Build history of the part. All positions in model axes, mm. Give positions to 0.01 mm unless a question says otherwise; leave off trailing zeros. Order: outer loops, then holes, each group sorted by start corner. A loop starts at its lowest first (then second) coordinate and runs counter-clockwise, first axis right, second up. Notation, with made-up numbers: (-36.75, 44.25) - (-21.75, 44.25) arc R19 ccw to (-21.75, 54.25) - close; hole circle Ø7 at (61.5, -17.5). An arc over 180 degrees is marked (long way). Write each question's results on one line, items separated by ' | '. Start each with the question number.
from build123d import *

# Parameters (mm, degrees)
SKETCH1_W           = 210
SKETCH1_H           = 60.3421622
SKETCH1_R           = 1.25
SKETCH1_R_2         = 2.5
SKETCH1_R_3         = 3.75
SKETCH1_R_4         = 5
SKETCH1_R_5         = 6.25
SKETCH1_R_6         = 7.5
SKETCH1_R_7         = 8.75
SKETCH1_R_8         = 10
SKETCH1_R_9         = 11.25
SKETCH1_R_10        = 12.5
SKETCH1_R_11        = 13.75
BOSS_EXTRUDE1_DEPTH = 10


with BuildPart() as part:
    # Sketch1 → Boss-Extrude1 (new body)
    with BuildSketch(Plane(origin=(0, 0, 0), x_dir=(1, 0, 0), z_dir=(0, 1, 0))):
        with Locations((93.75, -15.1710811)):
            Rectangle(SKETCH1_W, SKETCH1_H)
        Circle(SKETCH1_R, mode=Mode.SUBTRACT)
        with Locations((23.75, 0)):
            Circle(SKETCH1_R_2, mode=Mode.SUBTRACT)
        with Locations((50, 0)):
            Circle(SKETCH1_R_3, mode=Mode.SUBTRACT)
        with Locations((78.75, 0)):
            Circle(SKETCH1_R_4, mode=Mode.SUBTRACT)
        with Locations((110, 0)):
            Circle(SKETCH1_R_5, mode=Mode.SUBTRACT)
        with Locations((143.75, 0)):
            Circle(SKETCH1_R_6, mode=Mode.SUBTRACT)
        with Locations((180, 0)):
            Circle(SKETCH1_R_7, mode=Mode.SUBTRACT)
        with Locations((178.75, -25.3421622)):
            Circle(SKETCH1_R_8, mode=Mode.SUBTRACT)
        with Locations((125.831772041, -25.3421622)):
            Circle(SKETCH1_R_9, mode=Mode.SUBTRACT)
        with Locations((70.418227959, -25)):
            Circle(SKETCH1_R_10, mode=Mode.SUBTRACT)
        with Locations((12.5, -25)):
            Circle(SKETCH1_R_11, mode=Mode.SUBTRACT)
    extrude(amount=BOSS_EXTRUDE1_DEPTH)


solid = part.part
Item 1: Probe line 1 along X through (y, z) = (3, 25); line 2 along X through (y, z) = (3, 22.5); line 3 along Z through (x, y) = (50, 3.25). List the from-to ranges inside material, lowest first. Write a range as from..to.
Item 2: Two-plate mould, pull along Z, no slides. Class faces 1 (the flat face through (92, 5, 45.342)), 2 (the cylindrical face through (18.84, 4.93, 37.2)), 3 (the flat face through (-11.25, 5, 16)): +Z half, -Z half, draft (parallel to the pull), parting line (faces both ways), or undercut.
Item 3: Cut at B-B, the plane z = 30. List the corners of the cut face in (x, y).
Item 4: Cut at A-A, the plane x = 110. List the corners of the cut face in (y, z).
Item 5: Cut at C-C, the plane x = 180. List the corners of the cut face in (y, z), then the cut area to 3 significant figures.
Item 6: Flat gauge pin, fed straight in: pin 1 Ø2 at (x, z) = (0, 0) entering from +Y. Where does the tip first touch, or does it go through?
Item 7: Cut at D-D, the plane y = 5.5. Count the separate pieces of the cut face and the enclosed holes in it, then the cut area to 3 significant figures.
Values found:
1) line 1: x = -11.25..-1.25, 26.25..57.92, 82.92..114.59, 137.08..168.76, 188.74..198.75 | line 2: x = -11.25..-1.02, 26.02..58.17, 82.67..114.95, 136.72..169.16, 188.34..198.75 | line 3: z = -15..-3.75, 3.75..45.34
2) face 1: +Z half | face 2: undercut | face 3: draft
3) outline: (-11.25, 0) - (-0.31, 0) - (-0.31, 10) - (-11.25, 10) - close; (25.31, 0) - (58.96, 0) - (58.96, 10) - (25.31, 10) - close; (81.87, 0) - (115.59, 0) - (115.59, 10) - (81.87, 10) - close; (136.07, 0) - (169.9, 0) - (169.9, 10) - (136.07, 10) - close; (187.6, 0) - (198.75, 0) - (198.75, 10) - (187.6, 10) - close
4) outline: (0, -15) - (10, -15) - (10, -6.25) - (0, -6.25) - close; (0, 6.25) - (10, 6.25) - (10, 45.34) - (0, 45.34) - close
5) outline: (0, -15) - (10, -15) - (10, -8.75) - (0, -8.75) - close; (0, 8.75) - (10, 8.75) - (10, 15.42) - (0, 15.42) - close; (0, 35.26) - (10, 35.26) - (10, 45.34) - (0, 45.34) - close | area: 230 mm2
6) pin 1: passes through
7) separate pieces: 1 | enclosed holes: 11 | area: 10,200 mm2
